Autodesk Inventor part; units mm, degrees
ref_plane "YZ Plane" through (0, 0, 0) normal (1, 0, 0) x (0, 1, 0)
ref_plane "XZ Plane" through (0, 0, 0) normal (0, 1, 0) x (-1, 0, 0)
ref_plane "XY Plane" through (0, 0, 0) normal (0, 0, 1) x (1, 0, 0)
sketch "Sketch1" plane through (0, 0, 0) normal (0, 1, 0) x (-1, 0, 0)
  line L0 (-8, 7.5) -> (8, 7.5)
  line L1 (8, 7.5) -> (8, -7.5)
  line L2 (8, -7.5) -> (-8, -7.5)
  line L3 (-8, -7.5) -> (-8, 7.5)
  line L4 (-8, 7.5) -> (8, -7.5) construction
  line L5 (8, 7.5) -> (-8, -7.5) construction
  point P0 (0, 0)
  dimension "d0" = 16
  dimension "d1" = 15
extrude "Extrusion1" add sketch "Sketch1" against normal blind 2
sketch "Sketch2" plane through (-8, 0, 5.5) normal (0, 0, 1) x (1, 0, 0)
  line L0 (16, 0) -> (0, 0)
  line L1 (0, 0) -> (0, -18)
  line L2 (0, -18) -> (16, -18)
  line L3 (16, -18) -> (16, 0)
edge flange "Flange1" height 18 angle 90 thickness 2 bend radius 2 thickness toward (0, 0, 1) relief tear relief width 2 relief depth 1 edges at (0, -2, 7.5) wall of the first edge with corners at (8, 0, 5.5) (-8, 0, 5.5) (-8, -18, 5.5) (8, -18, 5.5)
bend "Bend1"
corner "Corner1"
sketch "Sketch3" plane through (8, -18, 5.5) normal (0, 0, -1) x (-1, 0, 0)
  line L0 (16, 14) -> (0, 14)
  line L1 (0, 14) -> (0, 0)
  line L2 (0, 0) -> (16, 0)
  line L3 (16, 14) -> (16, 0)
  line L4 (16, 14) -> (0, 14)
  line L5 (16, 16) -> (16, 14)
  line L6 (0, 16) -> (16, 16)
  line L7 (0, 16) -> (0, 14)
  line L8 (0, 0) -> (16, 0)
  line L9 (8, 0) -> (8, 16) construction
  point P0 (8, 18)
  point P1 (8, 8)
  dimension "d15" = 8
hole "Hole1" at (0, -10, 5.5) direction (0, 0, 1) diameter 10 end through all
equation "\"d21\" = Thickness"
equation "\"d4\" = Thickness"
equation "\"d5\" = BendReliefWidth"
equation "\"d6\" = BendReliefDepth"
equation "\"d7\" = MinimumRemnant"
equation "\"d8\" = TransitionRadius"
equation "\"d11\" = BendRadius"
equation "\"d12\" = CornerReliefSize"
equation "\"d13\" = GapSize"
equation "\"d14\" = JacobiRadiusSize"
equation "\"BendRadius\" = Thickness"
equation "\"BendReliefWidth\" = Thickness"
equation "\"BendReliefDepth\" = 0.5 * Thickness"
equation "\"CornerReliefSize\" = 4 * Thickness"
equation "\"MinimumRemnant\" = 2 * Thickness"
equation "\"TransitionRadius\" = BendRadius"
equation "\"JacobiRadiusSize\" = BendRadius"
equation "\"GapSize\" = Thickness"
properties part number "WheelMount No Motor"
Input: part model. Units: mm. Frame: model coordinates. A direction names the side the tool comes from. Give positions to 0.01 mm unless a question says otherwise; leave off trailing zeros. Loops run counter-clockwise (first coordinate to the right, second up) from the corner with the lowest first, then second, coordinate; pieces in that order, holes last. Notation, with made-up numbers: M -28.5,72 L 10.5,72 A22 cw 10.5,103 Z; hole C -36,13.5 d9. An arc over 180 degrees is marked long. Use CSV: the item, a comma, the result in double quotes.
(1) Section B-B, the plane x = 0. Return loops of the section in (y, z), plus the area to 3 significant figures.
Outcome:
outline,"M -18,5.5 L -15,5.5 L -15,7.5 L -18,7.5 Z; M -5,5.5 L -4,5.5 A2 cw -2,3.5 L -2,-7.5 L 0,-7.5 L 0,3.5 A4 ccw -4,7.5 L -5,7.5 Z"
area,"39.4 mm²"
(2) Pin query (flat end, axial travel): P1, Ø6, axis at x = 0, y = -10, coming from the -Z side; P2, Ø5, axis at x = 3.5, y = -5.5, coming from the -Z side; P3, Ø5.5, axis at x = -3.5, z = -2, coming from the -Y side; P4, Ø7, axis at x = 1.5, y = -13.5, coming from the -Z side. Return the tip coordinate at first contact, or that it passes through.
Outcome:
P1,"passes through"
P2,"stops at z = 5.23"
P3,"stops at y = -2"
P4,"stops at z = 5.5"
(3) Set-up query: faces 4 (the face through (0, 0, -2)), 5 (the face through (0, -16, 5.5)). Return all of +Z, -Z, +X, -X, +Y, -Y with unobstructed straight access to the full face (end or side cutting, diameter ignored); none if empty.
Outcome:
face 4,"+Z, -Z, +X, -X, +Y"
face 5,"-Z, +X, -X, -Y"
(4) Section A-A, the plane y = -10. Return loops of the section in (x, z), plus the area to 3 significant figures.
Outcome:
outline,"M -8,5.5 L -5,5.5 L -5,7.5 L -8,7.5 Z; M 5,5.5 L 8,5.5 L 8,7.5 L 5,7.5 Z"
area,"12.0 mm²"
(5) Material intervals for L1, parallel to X at y = -10, z = 6.45; L2, parallel to Y at x = 2.5, z = -2.25; L3, parallel to Z at x = -2.5, y = -15.5, sorted ascending. Write a range as [from, to].
Outcome:
L1,"x = [-8, -5], [5, 8]"
L2,"y = [-2, 0]"
L3,"z = [5.5, 7.5]"
(6) Pull-direction query (Y, two-part tool) for faces 1 (the face through (-8, -6, 6)), 2 (the face through (-0.112, -1.203, 6.359)), 3 (the face through (-1.5, -5.23, 6.51)); classes: pulls with the +Y half, pulls with the -Y half, needs draft (parallel to the pull), parting line crosses it, or undercut.
Outcome:
face 1,"needs draft"
face 2,"pulls with the +Y half"
face 3,"undercut"
(7) Section D-D, the plane y = -7.5. Return loops of the section in (x, z).
Outcome:
outline,"M -8,5.5 L -4.33,5.5 L -4.33,7.5 L -8,7.5 Z; M 4.33,5.5 L 8,5.5 L 8,7.5 L 4.33,7.5 Z"
(8) Section C-C, the plane x = -5.25. Return loops of the section in (y, z), plus the area to 3 significant figures.
Outcome:
outline,"M -18,5.5 L -4,5.5 A2 cw -2,3.5 L -2,-7.5 L 0,-7.5 L 0,3.5 A4 ccw -4,7.5 L -18,7.5 Z"
area,"59.4 mm²"
